Autodesk Inventor part; units mm, degrees
ref_plane "YZ Plane" through (0, 0, 0) normal (1, 0, 0) x (0, 1, 0)
ref_plane "XZ Plane" through (0, 0, 0) normal (0, 1, 0) x (-1, 0, 0)
ref_plane "XY Plane" through (0, 0, 0) normal (0, 0, 1) x (1, 0, 0)
sketch "Sketch1" plane through (0, 0, 0) normal (0, 1, 0) x (-1, 0, 0)
  line L0 (0, 0) -> (38.1, 0)
  line L1 (38.1, 0) -> (38.1, -50.8)
  line L2 (38.1, -50.8) -> (0, -50.8)
  line L3 (0, -50.8) -> (0, 0)
  line L4 (38.1, -50.8) -> (33.02, -50.8)
  line L5 (33.02, -50.8) -> (33.02, 0)
  line L6 (33.02, 0) -> (38.1, 0)
  line L7 (38.1, 0) -> (38.1, -50.8)
  line L8 (0, -50.8) -> (5.08, -50.8)
  line L9 (5.08, -50.8) -> (5.08, 0)
  line L10 (5.08, 0) -> (0, 0)
  line L11 (0, 0) -> (0, -50.8)
  dimension "d0" = 38.1
  dimension "d1" = 50.8
  dimension "d2" = 5.08
  dimension "d3" = 5.08
extrude "Extrusion1" add sketch "Sketch1" along normal blind 25.4 contours L0 L9 L2 L3 | L0 L1 L2 L5
extrude "Extrusion2" add sketch "Sketch1" against normal blind 5.08
sketch "Sketch2" plane through (0, 25.4, 0) normal (1, 0, 0) x (0, 0, -1)
  line L0 (50.8, 0) -> (0, 0)
  line L1 (25.4, 0) -> (25.4, -12.7)
  point P0 (0, -25.4)
  dimension "d8" = 12.7
hole "Hole1" at (0, 12.7, -25.4) direction (-1, 0, 0) diameter 6.7564 end through all
properties part number "Clip for 1 in 8020"
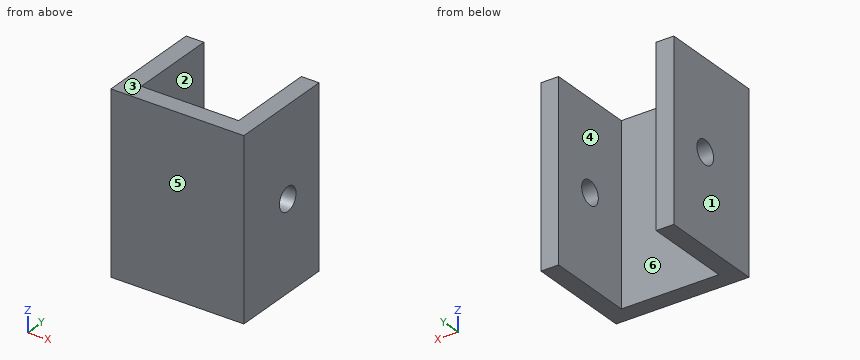
Design review of the part built by this model. Coordinates are the model's own, in mm. Face numbers are marked on the shaded views. A direction names the side the tool comes from. Round coordinates to 2 decimals unless told otherwise and drop trailing zeros. Loops run counter-clockwise (first coordinate to the right, second up) from the corner with the lowest first, then second, coordinate; pieces in that order, holes last. Notation, with made-up numbers: M -17,88.25 L 27,88.25 A16 cw 27,118.25 Z; hole C 56,56 d7. An arc over 180 degrees is marked long. Answer as a JSON object with one key per item and string values.
Item 1: We need section D-D on z = -15. Give the boundary of the cut face in (x, y), and give its area (3 significant figures).
Answer sheet:
{"outline": "M -38.1,-5.08 L 0,-5.08 L 0,25.4 L -5.08,25.4 L -5.08,0 L -33.02,0 L -33.02,25.4 L -38.1,25.4 Z", "area": "452 mm^2"}
Item 2: We need section A-A on y = 12.7. Give the boundary of the cut face in (x, z), and give its area (3 significant figures).
Answer sheet:
{"outline": "M -38.1,-50.8 L -33.02,-50.8 L -33.02,-28.78 L -38.1,-28.78 Z; M -38.1,-22.02 L -33.02,-22.02 L -33.02,0 L -38.1,0 Z; M -5.08,-50.8 L 0,-50.8 L 0,-28.78 L -5.08,-28.78 Z; M -5.08,-22.02 L 0,-22.02 L 0,0 L -5.08,0 Z", "area": "447 mm^2"}
Item 3: The part is to be moulded in two halves that separate along X. For the marked faces 1, 2, 3 and 4, say which applies: pulls with the +X half, pulls with the -X half, needs draft (parallel to the pull), parting line crosses it, or undercut.
Answer sheet:
{"face 1": "pulls with the -X half", "face 2": "undercut", "face 3": "needs draft", "face 4": "undercut"}
Item 4: Clearance check with flat-ended pins moving along their axes: P1, Ø6, axis at y = 12.7, z = -25.4, coming from the -X side (1 decimal); P2, Ø9, axis at y = 12.7, z = -25.4, coming from the +X side; P3, Ø8.5, axis at x = -17, z = -31.5, coming from the +Y side. State where each tip first meets the part, or that it passes through.
Answer sheet:
{"P1": "passes through", "P2": "stops at x = 0", "P3": "stops at y = 0"}
Item 5: We need section C-C on y = 6. Give the boundary of the cut face in (x, z), and give its area (3 significant figures).
Answer sheet:
{"outline": "M -38.1,-50.8 L -33.02,-50.8 L -33.02,0 L -38.1,0 Z; M -5.08,-50.8 L 0,-50.8 L 0,0 L -5.08,0 Z", "area": "516 mm^2"}
Item 6: Machinability: for the marked faces 5 and 6, which of the approach directions +Z, -Z, +X, -X, +Y, -Y give a long, thin tool a straight path to every point of the face, cutting with its end or side? Answer none if there is none.
Answer sheet:
{"face 5": "+Z, -Z, +X, -X, -Y", "face 6": "+Z, -Z, +Y"}
Item 7: We need section B-B on z = -25.4. Give the boundary of the cut face in (x, y), and give its area (3 significant figures).
Answer sheet:
{"outline": "M -38.1,-5.08 L 0,-5.08 L 0,9.32 L -5.08,9.32 L -5.08,0 L -33.02,0 L -33.02,9.32 L -38.1,9.32 Z; M -38.1,16.08 L -33.02,16.08 L -33.02,25.4 L -38.1,25.4 Z; M -5.08,16.08 L 0,16.08 L 0,25.4 L -5.08,25.4 Z", "area": "383 mm^2"}
Item 8: Wall thickness on L1, parallel to X at y = 9.5, z = -41.5; L2, parallel to Z at x = -1.5, y = 13; L3, parallel to Y at x = -3.3, z = -25.4: over which ranges is each line inside the solid? List them lowest first. Write a range as from..to.
Answer sheet:
{"L1": "x = -38.1..-33.02, -5.08..0", "L2": "z = -50.8..-28.76, -22.04..0", "L3": "y = -5.08..9.32, 16.08..25.4"}
